Check sheet for the modelled part. Datum: model origin and axes. Units: mm. A direction names the side the tool comes from. Coordinates: 2 decimals unless noted, no trailing zeros. Order: outer loops, then holes, each group sorted by start corner. A loop starts at its lowest first (then second) coordinate and runs counter-clockwise, first axis right, second up. Notation, with made-up numbers: M 59,84.25 L 78,84.25 A24 ccw 78,110.25 Z; hole C 39.5,40 d10. An arc over 180 degrees is marked long. Answer in a Markdown table with one row per item. Add a question column.
from build123d import *

# Parameters (mm, degrees)
SKETCH002_R  = 12
PAD001_DEPTH = 30
SKETCH_R     = 20
PAD_DEPTH    = 30


with BuildPart() as obj1:
    # Sketch002 → Pad001 (new body, symmetric)
    with BuildSketch(Plane.XZ):
        with BuildLine():
            Line((-30, 14), (-30, 10))
            Line((-30, 10), (42, 10))
            ThreePointArc((42, 4), (45, 7), (42, 10))
            Line((42, 4), (-30, 4))
            Line((-30, 4), (-30, 0))
            Line((-30, 0), (60, 0))
            ThreePointArc((60, 0), (72.369317, 23.485281), (46.005715, 20.4))
            ThreePointArc((36.676192, 14), (42.333047, 15.753789), (46.005715, 20.4))
            Line((36.676192, 14), (-30, 14))
        make_face()
        with Locations((60, 15)):
            Circle(SKETCH002_R, mode=Mode.SUBTRACT)
    extrude(amount=PAD001_DEPTH, both=True)


with BuildPart() as obj2:
    # Sketch → Pad (new body)
    with BuildSketch(Plane.XY):
        with BuildLine():
            Line((75, 25), (75, 20))
            Line((75, 20), (37, 20))
            ThreePointArc((37, 20), (33.464466, 18.535534), (32, 15))
            Line((32, 15), (32, -15))
            ThreePointArc((32, -15), (33.464466, -18.535534), (37, -20))
            Line((37, -20), (75, -20))
            Line((75, -20), (75, -25))
            Line((19.364917, -25), (75, -25))
            ThreePointArc((19.364917, -25), (16.864917, -25.317542), (14.523688, -26.25))
            ThreePointArc((14.523688, 26.25), (-30, 0), (14.523688, -26.25))
            ThreePointArc((14.523688, 26.25), (16.864917, 25.317542), (19.364917, 25))
            Line((75, 25), (19.364917, 25))
        make_face()
        Circle(SKETCH_R, mode=Mode.SUBTRACT)
    extrude(amount=PAD_DEPTH)

    # Boolean: intersect obj1
    add(obj1.part, mode=Mode.INTERSECT)


solid = obj2.part
1. Section check D-D on y = -23. Enter the section's corners in (x, z).
2. Release check for a two-part mould opening along Y. For faces 1 (the cylindrical face through (-29.987, 0.872, 1.972)), 2 (the flat face through (32, 0, 12)), 3 (the cylindrical face through (16.831, 25.326, 1.972)) record: released by +Y, released by -Y, zero draft, split by the parting line, or undercut.
3. Section check A-A on y = 0. Enter the section's corners in (x, z), then the cut area to 3 significant figures.
4. Go/stop test with flat-tipped pins: pin 1 Ø2 at (y, z) = (4, 2) entering from +X; pin 2 Ø18 at (x, y) = (-12, 10.5) entering from +Z; pin 3 Ø6 at (x, z) = (-13.5, 12.5) entering from +Y. Record where each tip stops, or that it passes through.
5. Section check C-C on z = 7. Enter the section's corners in (x, y), then the cut area to 3 significant figures.
6. Scan lines: line 1 (Y direction, x = 47, z = 20); line 2 (Z direction, x = 60, y = 23.95); line 3 (Z direction, x = -19, y = 21). Record each from-to range of solid material in increasing order.
7. Section check B-B on z = 12.5. Enter the section's corners in (x, y).
8. Set-up check for faces 4 (the flat face through (47, -25, 10)), 5 (the flat face through (21, 0, 10)), 6 (the flat face through (49, -20, 8)): record each of +Z, -Z, +X, -X, +Y, -Y from which the full face is reachable in a straight line by a thin tool's end or side.
Result sheet:
| question | item | result |
|---|---|---|
| 1 | outline | M -19.26,0 L 60,0 A15 ccw long 46.01,20.4 A10 cw 36.68,14 L -19.26,14 L -19.26,10 L 42,10 A3 cw 42,4 L -19.26,4 Z; hole C 60,15 d24 |
| 2 | face 1 | split by the parting line |
| 2 | face 2 | undercut |
| 2 | face 3 | released by +Y |
| 3 | outline | M -30,0 L -20,0 L -20,4 L -30,4 Z; M -30,10 L -20,10 L -20,14 L -30,14 Z; M 20,0 L 32,0 L 32,4 L 20,4 Z; M 20,10 L 32,10 L 32,14 L 20,14 Z |
| 3 | area | 176 mm^2 |
| 4 | pin 1 | x = 32 |
| 4 | pin 2 | z = 14 |
| 4 | pin 3 | y = 28.1 |
| 5 | outline | M 45,-25 L 51.06,-25 L 51.06,-20 L 45,-20 Z; M 45,20 L 51.06,20 L 51.06,25 L 45,25 Z; M 68.94,-25 L 72.69,-25 L 72.69,-20 L 68.94,-20 Z; M 68.94,20 L 72.69,20 L 72.69,25 L 68.94,25 Z |
| 5 | area | 98.0 mm^2 |
| 6 | line 1 | -25 to -20, 20 to 25 |
| 6 | line 2 | 0 to 3, 27 to 30 |
| 6 | line 3 | 0 to 4, 10 to 14 |
| 7 | outline | M 14.52,-26.25 A10 cw 19.36,-25 L 48.26,-25 L 48.26,-20 L 37,-20 A5 cw 32,-15 L 32,15 A5 cw 37,20 L 48.26,20 L 48.26,25 L 19.36,25 A10 cw 14.52,26.25 A30 ccw long Z; M 71.74,-25 L 74.79,-25 L 74.79,-20 L 71.74,-20 Z; M 71.74,20 L 74.79,20 L 74.79,25 L 71.74,25 Z; hole C 0,0 d40 |
| 8 | face 4 | +Z, -Z, +X, -Y |
| 8 | face 5 | -X, +Y, -Y |
| 8 | face 6 | +Z, -Z, +X |
